Geometry: see drawing. Coordinates: mm, zero at the bounding-box minimum. A direction names the side the tool comes from. Give positions to 0.01 mm unless a question says otherwise; leave off trailing zeros. Loops run counter-clockwise (first coordinate to the right, second up) from the corner with the lowest first, then second, coordinate; pieces in that order, holes last. Notation, with made-up numbers: M -17.5,-15.75 L 27.5,-15.75 A10 ccw 27.5,-9.75 Z; hole C 18,78 d10. An arc over 180 degrees is marked long. Return JSON: item names as keys, results as strings. Group by question number.
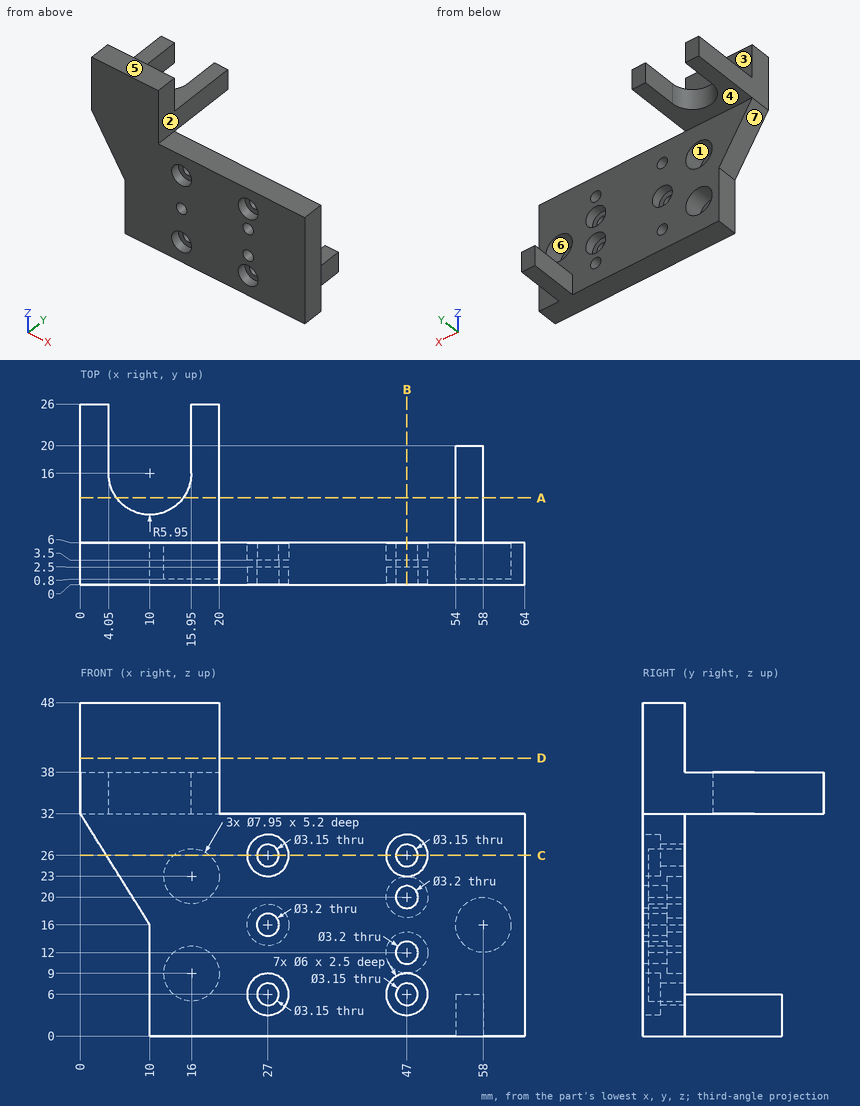
Item 1: Section A-A, the plane y = 12.5. Return loops of the section in (x, z), then the cut area to 3 significant figures.
Item 2: Material intervals for line 1 (Z direction, x = 27, y = 0.8); line 2 (Z direction, x = 47, y = 4.95) (3 decimals); line 3 (X direction, y = 4.85, z = 16) (3 decimals), sorted ascending. Write a range as from..to.
Item 3: Pull-direction query (X, two-part tool) for the marked faces 5, 6 and 7; classes: pulls with the +X half, pulls with the -X half, needs draft (parallel to the pull), parting line crosses it, or undercut.
Item 4: Section B-B, the plane x = 47. Give the number of separate pieces and of enclosed holes in the cut face, then the cut area to 4 significant figures.
Item 5: First-contact query: pin 1 Ø8 at (x, z) = (36.5, 21) entering from +Y; pin 2 Ø3 at (x, z) = (47, 6) entering from -Y; pin 3 Ø4 at (y, z) = (4.5, 41.5) entering from +X; pin 4 Ø5.5 at (x, z) = (47, 20) entering from -Y. Flat tips, straight axial feed; report the tip coordinate or a pass-through.
Item 6: Section D-D, the plane z = 40. Return loops of the section in (x, y), then the cut area to 3 significant figures.
Item 7: Section C-C, the plane z = 26. Return loops of the section in (x, y) (3 decimals).
Item 8: Reachability of the marked faces 1, 2, 3 and 4 from +Z, -Z, +X, -X, +Y, -Y: full face, straight path, thin tool, end or side. Return the list, or none.
Answer below:
{
 "1": {"outline": "M 0,32 L 5.19,32 L 5.19,38 L 0,38 Z; M 14.81,32 L 20,32 L 20,38 L 14.81,38 Z; M 54,0 L 58,0 L 58,6 L 54,6 Z", "area": "86.3 mm^2"},
 "2": {"line 1": "0..3, 9..14.4, 17.6..23, 29..32", "line 2": "0..4.425, 7.575..9, 15..17, 23..24.425, 27.575..32", "line 3": "10..24, 30..54.025, 61.975..64"},
 "3": {"face 5": "needs draft", "face 6": "undercut", "face 7": "pulls with the -X half"},
 "4": {"separate pieces": "5", "enclosed holes": "0", "area": "87.55 mm^2"},
 "5": {"pin 1": "y = 6", "pin 2": "through", "pin 3": "x = 20", "pin 4": "y = 0"},
 "6": {"outline": "M 0,0 L 20,0 L 20,6 L 0,6 Z", "area": "120 mm^2"},
 "7": {"outline": "M 3.75,0 L 24,0 L 24,2.5 L 25.425,2.5 L 25.425,6 L 18.608,6 L 18.608,0.8 L 13.392,0.8 L 13.392,6 L 3.75,6 Z; M 28.575,2.5 L 30,2.5 L 30,0 L 44,0 L 44,2.5 L 45.425,2.5 L 45.425,6 L 28.575,6 Z; M 48.575,2.5 L 50,2.5 L 50,0 L 64,0 L 64,6 L 48.575,6 Z"},
 "8": {"face 1": "+Y", "face 2": "+Z, +X, +Y, -Y", "face 3": "+Z, +X, -X, +Y", "face 4": "-Z, +X, -X, +Y"}
}
